Geometry: see drawing. Coordinates: mm, zero at the bounding-box minimum. A direction names the side the tool comes from. Give positions to 0.01 mm unless a question says otherwise; leave off trailing zeros. Order: outer loops, then holes, each group sorted by start corner. A loop starts at its lowest first (then second) coordinate and runs counter-clockwise, first axis right, second up. Notation, with made-up numbers: M 25.25,28 L 71.25,28 A20 ccw 71.25,42 Z; hole C 32,3 d2. An arc over 180 degrees is marked long. Use a Markdown table: item, result.
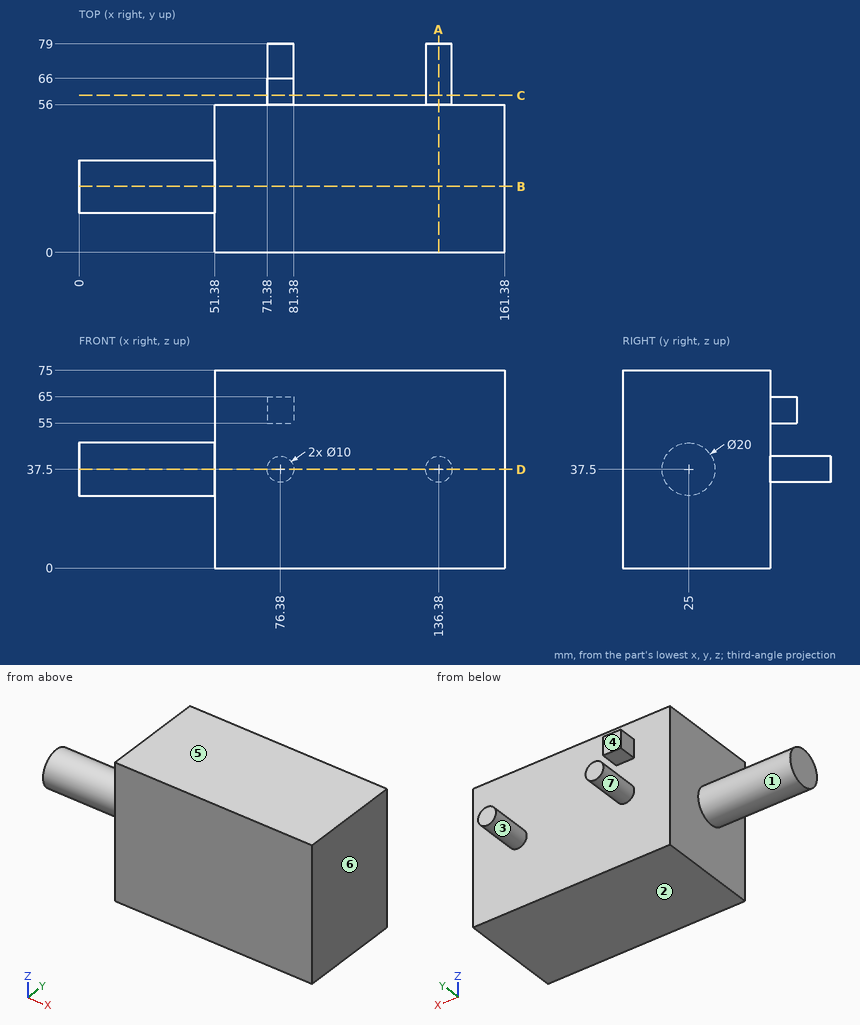
1) Material intervals for line 1 (X direction, y = 53, z = 35); line 2 (Y direction, x = 148, z = 25); line 3 (Y direction, x = 24.5, z = 44.5), sorted ascending. Write a range as from..to.
Response values:
| item | result |
|---|---|
| line 1 | x = 51.38..161.38 |
| line 2 | y = 0..56 |
| line 3 | y = 17.86..32.14 |
2) Reachability of the marked faces 1, 2, 3 and 4 from +Z, -Z, +X, -X, +Y, -Y: full face, straight path, thin tool, end or side. Return the list, or none.
Response values:
| item | result |
|---|---|
| face 1 | -X |
| face 2 | -Z, +X, -X, +Y, -Y |
| face 3 | +Y |
| face 4 | +Z, +X, -X, +Y |
3) First-contact query: pin 1 Ø10 at (y, z) = (26, 32.5) entering from -X; pin 2 Ø11 at (x, y) = (76.5, 63) entering from -Z; pin 3 Ø12 at (x, z) = (128, 25) entering from +Y; pin 4 Ø6 at (y, z) = (10.5, 29) entering from -X. Flat tips, straight axial feed; report the tip coordinate or a pass-through.
Response values:
| item | result |
|---|---|
| pin 1 | stops at x = 0 |
| pin 2 | stops at z = 32.5 |
| pin 3 | stops at y = 56 |
| pin 4 | stops at x = 51.38 |
4) Cut plane A-A on x = 136.38. Return loops of the section in (y, z).
Response values:
| item | result |
|---|---|
| outline | M 0,0 L 56,0 L 56,32.5 L 79,32.5 L 79,42.5 L 56,42.5 L 56,75 L 0,75 Z |
5) Mould query, pull axis X, two halves, no side actions, for the marked faces 5, 6 and 7. Classes: released by +X, released by -X, zero draft, split by the parting line, or undercut.
Response values:
| item | result |
|---|---|
| face 5 | zero draft |
| face 6 | released by +X |
| face 7 | undercut |
6) Cut plane C-C on y = 59.5. Return loops of the section in (x, z), and give its area (3 significant figures).
Response values:
| item | result |
|---|---|
| outline | C 76.38,37.5 d10; M 71.38,55 L 81.38,55 L 81.38,65 L 71.38,65 Z; C 136.38,37.5 d10 |
| area | 257 mm² |
7) Cut plane D-D on z = 37.5. Return loops of the section in (x, y), and give its area (3 significant figures).
Response values:
| item | result |
|---|---|
| outline | M 0,15 L 51.38,15 L 51.38,0 L 161.38,0 L 161.38,56 L 141.38,56 L 141.38,79 L 131.38,79 L 131.38,56 L 81.38,56 L 81.38,79 L 71.38,79 L 71.38,56 L 51.38,56 L 51.38,35 L 0,35 Z |
| area | 7,650 mm² |
8) Cut plane B-B on y = 25. Return loops of the section in (x, z), and give its area (3 significant figures).
Response values:
| item | result |
|---|---|
| outline | M 0,27.5 L 51.38,27.5 L 51.38,0 L 161.38,0 L 161.38,75 L 51.38,75 L 51.38,47.5 L 0,47.5 Z |
| area | 9,280 mm² |
